Source: CAD feature listing. Evaluate the final solid. Frame: model axes, mm. Face numbers are marked on the shaded views. A direction names the side the tool comes from. Coordinates: 2 decimals unless noted, no trailing zeros. Order: outer loops, then holes, each group sorted by start corner. A loop starts at its lowest first (then second) coordinate and runs counter-clockwise, first axis right, second up.
```python
from build123d import *

# Parameters (mm, degrees)
SKETCH1_R           = 0.815
BOSS_EXTRUDE1_DEPTH = 1
SKETCH2_W           = 1.01
SKETCH2_H           = 4
CUT_EXTRUDE1_DEPTH  = 1.01


with BuildPart() as part:
    # Sketch1 → Boss-Extrude1 (new, symmetric)
    with BuildSketch(Plane.XY):
        with BuildLine():
            Line((0, 0), (0, 8))
            ThreePointArc((0, 8), (1.757359313, 12.242640687), (6, 14))
            Line((6, 14), (11.25, 14))
            Line((11.25, 14), (11.25, 10))
            Line((11.25, 10), (8, 10))
            ThreePointArc((8, 10), (5.171572875, 8.828427125), (4, 6))
            Line((4, 6), (4, 0))
            Line((4, 0), (0, 0))
        make_face()
        with Locations((9.56, 12)):
            Circle(SKETCH1_R, mode=Mode.SUBTRACT)
    extrude(amount=BOSS_EXTRUDE1_DEPTH, both=True)

    # Sketch2 → Cut-Extrude1 (cut)
    with BuildSketch(Plane(origin=(11.25, 0, 0), x_dir=(0, 0, -1), z_dir=(1, 0, 0))):
        with Locations((0, 12)):
            Rectangle(SKETCH2_W, SKETCH2_H)
    extrude(amount=-CUT_EXTRUDE1_DEPTH, mode=Mode.SUBTRACT)


solid = part.part
```
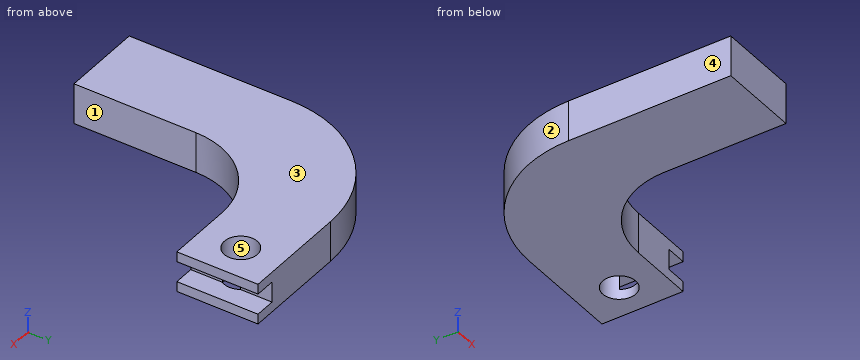
Q1. Set-up query: the marked faces 1 and 2. Return all of +Z, -Z, +X, -X, +Y, -Y with unobstructed straight access to the full face (end or side cutting, diameter ignored); none if empty.
Solutions:
face 1: +Z, -Z, +X, -Y
face 2: +Z, -Z, -X, +Y
Q2. Material intervals for line 1 along Y through (x, z) = (9.5, -0.9); line 2 along X through (y, z) = (6, 0.45); line 3 along Z through (x, y) = (10.75, 12.5) (3 decimals), sorted ascending.
Solutions:
line 1: y = 10 to 11.19, 12.81 to 14
line 2: x = 0 to 4
line 3: z = -1 to -0.505, 0.505 to 1
Q3. Section query D-D on z = 0.1. Output: boundary loops of the cut face in (x, y) (3 decimals).
Solutions:
outline: (0, 0) - (4, 0) - (4, 6) arc R4 cw to (8, 10) - (10.24, 10) - (10.24, 11.551) arc R0.815 cw (long way) to (10.24, 12.449) - (10.24, 14) - (6, 14) arc R6 ccw to (0, 8) - close
Q4. Section query C-C on z = -0.7. Output: boundary loops of the cut face in (x, y) (3 decimals).
Solutions:
outline: (0, 0) - (4, 0) - (4, 6) arc R4 cw to (8, 10) - (11.25, 10) - (11.25, 14) - (6, 14) arc R6 ccw to (0, 8) - close; hole circle Ø1.63 at (9.56, 12)
Q5. Section query B-B on y = 12. Output: boundary loops of the cut face in (x, z) (3 decimals).
Solutions:
outline: (1.528, -1) - (8.745, -1) - (8.745, 1) - (1.528, 1) - close; (10.375, -1) - (11.25, -1) - (11.25, -0.505) - (10.375, -0.505) - close; (10.375, 0.505) - (11.25, 0.505) - (11.25, 1) - (10.375, 1) - close
Q6. Pin query (flat end, axial travel): P1, Ø1, axis at y = 2, z = -0.5, coming from the -X side. Return the tip coordinate at first contact, or that it passes through.
Solutions:
P1: stops at x = 0
Q7. Section query A-A on x = 9.56. Output: boundary loops of the cut face in (y, z) (3 decimals).
Solutions:
outline: (10, -1) - (11.185, -1) - (11.185, 1) - (10, 1) - close; (12.815, -1) - (14, -1) - (14, 1) - (12.815, 1) - close
Q8. Pull-direction query (X, two-part tool) for the marked faces 3, 4 and 5; classes: pulls with the +X half, pulls with the -X half, needs draft (parallel to the pull), parting line crosses it, or undercut.
Solutions:
face 3: needs draft
face 4: pulls with the -X half
face 5: undercut
